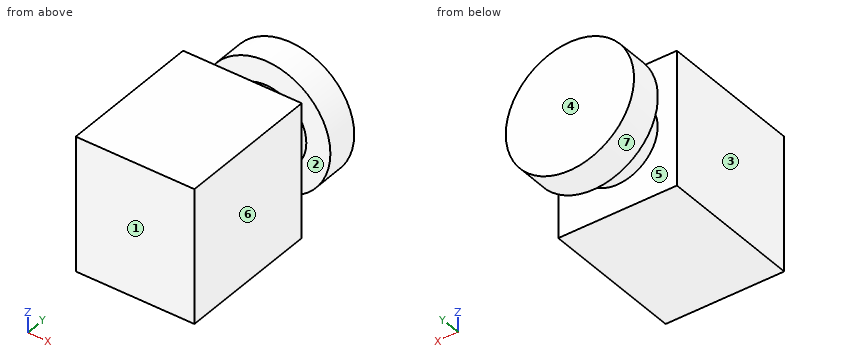
Autodesk Inventor part; units mm, degrees
ref_plane "YZ Plane" through (0, 0, 0) normal (1, 0, 0) x (0, 1, 0)
ref_plane "XZ Plane" through (0, 0, 0) normal (0, 1, 0) x (-1, 0, 0)
ref_plane "XY Plane" through (0, 0, 0) normal (0, 0, 1) x (1, 0, 0)
sketch "Sketch1" plane through (0, 0, 0) normal (0, 1, 0) x (-1, 0, 0)
  line L0 (-18.5, 21) -> (18.5, 21)
  line L1 (18.5, 21) -> (18.5, -21)
  line L2 (18.5, -21) -> (-18.5, -21)
  line L3 (-18.5, -21) -> (-18.5, 21)
  line L4 (-18.5, 21) -> (18.5, -21) construction
  line L5 (18.5, 21) -> (-18.5, -21) construction
  point P0 (0, 0)
  dimension "d0" = 37
  dimension "d1" = 42
extrude "Extrusion1" add sketch "Sketch1" along normal blind 45
sketch "Sketch2" plane through (0, 45, 0) normal (0, 1, 0) x (1, 0, 0)
  circle A0 centre (0, 0) radius 12.5
  dimension "d4" = 25
extrude "Extrusion2" add sketch "Sketch2" along normal blind 10
sketch "Sketch3" plane through (0, 55, 0) normal (0, 1, 0) x (1, 0, 0)
  circle A0 centre (0, 0) radius 20
  dimension "d7" = 40
extrude "Extrusion3" add sketch "Sketch3" along normal blind 10
properties part number "emergency_stop"
Input: part model. Units: mm. Frame: model coordinates. Face numbers are marked on the shaded views. A direction names the side the tool comes from. Coordinates: 2 decimals unless noted, no trailing zeros. Loops run counter-clockwise (first coordinate to the right, second up) from the corner with the lowest first, then second, coordinate; pieces in that order, holes last.
(1) Pull-direction query (Y, two-part tool) for the marked faces 1, 2, 3 and 4; classes: released by +Y, released by -Y, zero draft, split by the parting line, or undercut.
(2) Section C-C on z = 13.5. Return the cut outline in (x, y), then the cut area to 3 significant figures.
(3) Section B-B on x = -14. Return the cut outline in (y, z).
(4) Section A-A on z = 0. Return the cut outline in (x, y).
(5) First-contact query: pin 1 Ø12.5 at (y, z) = (19, -8.5) entering from +X; pin 2 Ø8 at (x, z) = (8, -5.5) entering from -Y; pin 3 Ø5 at (y, z) = (38.5, 9) entering from -X; pin 4 Ø4 at (x, y) = (9, 52.5) entering from -Z. Flat tips, straight axial feed; report the tip coordinate or a pass-through.
(6) Section D-D on x = 0. Return the cut outline in (y, z).
(7) Material intervals for probe 1 along Y at (x, z) = (10.5, -12); probe 2 along X at (y, z) = (8.5, 13); probe 3 along Y at (x, z) = (13, -18), sorted ascending.
(8) Set-up query: the marked faces 5, 6 and 7. Return all of +Z, -Z, +X, -X, +Y, -Y with unobstructed straight access to the full face (end or side cutting, diameter ignored); none if empty.
Data:
1. face 1: released by -Y
1. face 2: undercut
1. face 3: zero draft
1. face 4: released by +Y
2. outline: (-18.5, 0) - (18.5, 0) - (18.5, 45) - (-18.5, 45) - close; (-14.76, 55) - (14.76, 55) - (14.76, 65) - (-14.76, 65) - close
2. area: 1,960 mm2
3. outline: (0, -21) - (45, -21) - (45, 21) - (0, 21) - close; (55, -14.28) - (65, -14.28) - (65, 14.28) - (55, 14.28) - close
4. outline: (-20, 55) - (-12.5, 55) - (-12.5, 45) - (-18.5, 45) - (-18.5, 0) - (18.5, 0) - (18.5, 45) - (12.5, 45) - (12.5, 55) - (20, 55) - (20, 65) - (-20, 65) - close
5. pin 1: stops at x = 18.5
5. pin 2: stops at y = 0
5. pin 3: stops at x = -18.5
5. pin 4: stops at z = -10.36
6. outline: (0, -21) - (45, -21) - (45, -12.5) - (55, -12.5) - (55, -20) - (65, -20) - (65, 20) - (55, 20) - (55, 12.5) - (45, 12.5) - (45, 21) - (0, 21) - close
7. probe 1: y = 0 to 45, 55 to 65
7. probe 2: x = -18.5 to 18.5
7. probe 3: y = 0 to 45
8. face 5: none
8. face 6: +Z, -Z, +X, -Y
8. face 7: +Y
